```python
from build123d import *

# Parameters (mm, degrees)
F1_DEPTH = 10.9
F0_R     = 12.75
F2_DEPTH = 52
F3_DEPTH = 2
F4_DEPTH = 2


with BuildPart() as f1:
    # F0 (on Top) → F1 (new body)
    with BuildSketch(Plane.XY):
        with BuildLine():
            ThreePointArc((10.749535, 10.1), (11.581471, 9.134113), (12.326901, 8.1))
            Line((12.326901, 8.1), (82.75, 8.1))
            Line((82.75, 8.1), (82.75, 10.1))
            Line((82.75, 10.1), (10.749535, 10.1))
        make_face()
        Polygon((82.75, 8.1), (82.75, 0), (82.75, -8.1), (82.75, -10.1), (84.75, -10.1), (84.75, 10.1), (82.75, 10.1), align=None)
        with BuildLine():
            Line((82.75, -8.1), (12.326901, -8.1))
            ThreePointArc((12.326901, -8.1), (11.581471, -9.134113), (10.749535, -10.1))
            Line((10.749535, -10.1), (82.75, -10.1))
            Line((82.75, -10.1), (82.75, -8.1))
        make_face()
    extrude(amount=F1_DEPTH)

    # F0 (on Top) → F2 (join)
    with BuildSketch(Plane.XY):
        with BuildLine():
            ThreePointArc((12.326901, -8.1), (14.131247, -4.227334), (14.75, 0))
            ThreePointArc((14.75, 0), (14.131247, 4.227334), (12.326901, 8.1))
            ThreePointArc((12.326901, 8.1), (11.581471, 9.134113), (10.749535, 10.1))
            ThreePointArc((10.749535, 10.1), (-14.75, 0), (10.749535, -10.1))
            ThreePointArc((10.749535, -10.1), (11.581471, -9.134113), (12.326901, -8.1))
        make_face()
        Circle(F0_R, mode=Mode.SUBTRACT)
    extrude(amount=F2_DEPTH)

    # F0 (on Top) → F3 (join)
    with BuildSketch(Plane.XY):
        with BuildLine():
            ThreePointArc((12.326901, 8.1), (14.131247, 4.227334), (14.75, 0))
            Line((14.75, 0), (82.75, 0))
            Line((82.75, 0), (82.75, 8.1))
            Line((82.75, 8.1), (12.326901, 8.1))
        make_face()
        with BuildLine():
            Line((82.75, 0), (14.75, 0))
            ThreePointArc((14.75, 0), (14.131247, -4.227334), (12.326901, -8.1))
            Line((12.326901, -8.1), (82.75, -8.1))
            Line((82.75, -8.1), (82.75, 0))
        make_face()
    extrude(amount=F3_DEPTH)

    # F0 (on Top) → F4 (join)
    with BuildSketch(Plane.XY):
        Circle(F0_R)
    extrude(amount=F4_DEPTH)


solid = f1.part
```
For this review, take the finished solid that the model builds, in its own axes (mm). A direction names the side the tool comes from. Coordinates: 2 decimals unless noted, no trailing zeros. Write each loop counter-clockwise with the first axis right and the second up, starting at its lowest first coordinate (ties: lowest second). Pieces come first, ordered by that corner, then holes. Notation, with made-up numbers: (45, 83.5) - (60, 83.5) arc R10 cw to (60, 90.5) - close; hole circle Ø9 at (51.25, -28.75). An arc over 180 degrees is marked (long way). Put each result on its own line as item: value.
1. Machinability: for faces 1 (the flat face through (84.75, 0, 5)), 2 (the flat face through (48, 10.1, 5)), 3 (the cylindrical face through (11.593, 9.12, 31.162)), 4 (the flat face through (47, -10.1, 5)), 5 (the flat face through (47, 8.1, 6)), which of the approach directions +Z, -Z, +X, -X, +Y, -Y give a long, thin tool a straight path to every point of the face, cutting with its end or side? Answer none if there is none.
Values found:
face 1: +Z, -Z, +X, +Y, -Y
face 2: +Z, -Z, +X, +Y
face 3: +Z, +X, +Y
face 4: +Z, -Z, +X, -Y
face 5: +Z
2. Wall thickness on probe 1 along Y at (x, z) = (0, 33); probe 2 along X at (y, z) = (5.25, 4); probe 3 along X at (y, z) = (-0.5, 32): over which ranges is each line inside the solid? List them lowest first.
Values found:
probe 1: -14.75 to -12.75, 12.75 to 14.75
probe 2: -13.78 to -11.62, 11.62 to 13.78, 82.75 to 84.75
probe 3: -14.74 to -12.74, 12.74 to 14.74
3. Add section B-B, the plane x = 0. Give the boundary of the cut face in (y, z).
Values found:
outline: (-14.75, 0) - (14.75, 0) - (14.75, 52) - (12.75, 52) - (12.75, 2) - (-12.75, 2) - (-12.75, 52) - (-14.75, 52) - close
4. Add section C-C, the plane z = 27. Give the boundary of the cut face in (x, y).
Values found:
outline: (10.75, -10.1) arc R14.75 ccw to (12.33, -8.1) arc R14.75 ccw to (14.75, 0) arc R14.75 ccw to (12.33, 8.1) arc R14.75 ccw to (10.75, 10.1) arc R14.75 ccw (long way) to start; hole circle Ø25.5 at (0, 0)
5. For pin 1 (10 mm diameter, centred on x = 57, z = 5, fed in from +Y); pin 2 (4 mm diameter, centred on y = -7, z = 29, fed in from +X); pin 3 (10 mm diameter, centred on x = 61, y = 3, fed in from +Z), all flat-tipped, find the tip position at first contact; note any pin that passes through.
Values found:
pin 1: y = 10.1
pin 2: x = 13.88
pin 3: z = 2
6. Add section D-D, the plane y = 3.5. Give the boundary of the cut face in (x, z).
Values found:
outline: (-14.33, 0) - (84.75, 0) - (84.75, 10.9) - (82.75, 10.9) - (82.75, 2) - (14.33, 2) - (14.33, 52) - (12.26, 52) - (12.26, 2) - (-12.26, 2) - (-12.26, 52) - (-14.33, 52) - close
7. Mouldability with a two-part tool opening along X and no side actions: class faces 6 (the flat face through (48, -8.1, 6)), 7 (the flat face through (34, 0, 0)), 8 (the cylindrical face through (11.57, -9.15, 31.16)), 9 (the cylindrical face through (-14.74, 0.49, 25.64)) as released by +X, released by -X, zero draft, split by the parting line, or undercut.
Values found:
face 6: undercut
face 7: zero draft
face 8: released by +X
face 9: split by the parting line
8. Add section A-A, the plane z = 8.5. Give the boundary of the cut face in (x, y), then the cut area to 3 significant figures.
Values found:
outline: (10.75, -10.1) - (84.75, -10.1) - (84.75, 10.1) - (10.75, 10.1) arc R14.75 ccw (long way) to start; hole circle Ø25.5 at (0, 0); hole (12.33, -8.1) - (82.75, -8.1) - (82.75, 8.1) - (12.33, 8.1) arc R14.75 cw to (14.75, 0) arc R14.75 cw to start
area: 498 mm²
